Could you check a few things on this model? Use its own coordinates, in mm. Face numbers are marked on the shaded views. A direction names the side the tool comes from. Round coordinates to 2 decimals unless told otherwise and drop trailing zeros. Loops run counter-clockwise (first coordinate to the right, second up) from the corner with the lowest first, then second, coordinate; pieces in that order, holes last. Notation, with made-up numbers: M 76,20 L 115,20 A20 cw 115,43 Z; hole C 30,-22.5 d2. An arc over 180 degrees is marked long. Return JSON: item names as keys, results as strings. Group by question number.
```python
from build123d import *

# Parameters (mm, degrees)
BOSS_EXTRUDE1_DEPTH     = 20
FILLET1_R               = 2
SHELL1_T                = -4
CUT_EXTRUDE1_DEPTH      = 43.708313008
CUT_EXTRUDE1_DEPTH_BACK = 43.708313008
SKETCH2_R               = 5


with BuildPart() as part:
    # Sketch1 → Boss-Extrude1 (new body)
    with BuildSketch(Plane.XY):
        with BuildLine():
            Line((-30, 20), (30, 20))
            ThreePointArc((30, 20), (31.414213562, 19.414213562), (32, 18))
            Line((32, 18), (32, -18))
            ThreePointArc((32, -18), (31.414213562, -19.414213562), (30, -20))
            Line((30, -20), (-30, -20))
            ThreePointArc((-30, -20), (-31.414213562, -19.414213562), (-32, -18))
            Line((-32, -18), (-32, 18))
            ThreePointArc((-32, 18), (-31.414213562, 19.414213562), (-30, 20))
        make_face()
    extrude(amount=BOSS_EXTRUDE1_DEPTH)

    # Fillet1
    fillet1_edges = [part.edges().sort_by_distance(p)[0] for p in [
        (0, -20, 0),
        (-31.414213562, -19.414213562, 0),
        (-32, 0, 0),
        (-31.414213562, 19.414213562, 0),
        (0, 20, 0),
        (31.414213562, 19.414213562, 0),
        (32, 0, 0),
        (31.414213562, -19.414213562, 0),
    ]]
    fillet(fillet1_edges, radius=FILLET1_R)

    # Shell1
    shell1_openings = [part.faces().sort_by_distance(p)[0] for p in [
        (0, 0, 20),
    ]]
    offset(amount=SHELL1_T, openings=shell1_openings, kind=Kind.INTERSECTION)

    # Sketch2 → Cut-Extrude1 (cut, two sides: drawn at the far end of the back side and taken through both)
    with BuildSketch(Plane(origin=(0, 0, 0), x_dir=(1, 0, 0), z_dir=(0, 1, 0)).offset(-CUT_EXTRUDE1_DEPTH_BACK)):
        with Locations((-16, -20)):
            Circle(SKETCH2_R)
        with Locations((16, -20)):
            Circle(SKETCH2_R)
    extrude(amount=CUT_EXTRUDE1_DEPTH + CUT_EXTRUDE1_DEPTH_BACK, mode=Mode.SUBTRACT)


solid = part.part
```
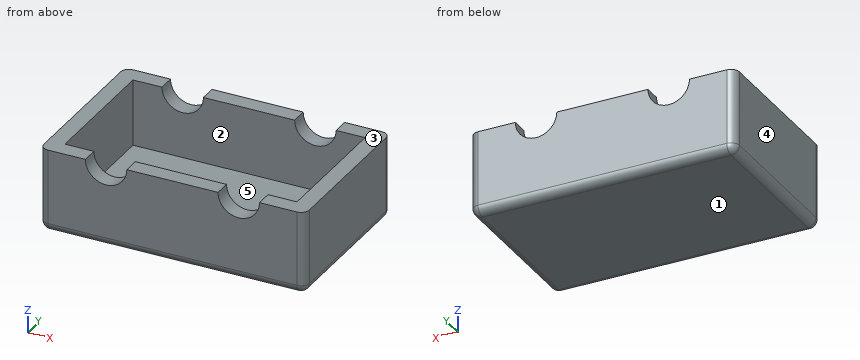
1. We'd pull the mould along X, two halves only. Please class the marked faces 3, 4 and 5: +X half, -X half, draft (parallel to the pull), parting line (faces both ways), or undercut.
2. I'm going to push a flat-ended pin straight in: pin 1 Ø9.5 at (x, y) = (-4, 1) entering from +Z. Where does the tip first touch, or does it pass through?
3. I need wall thicknesses on probe 1 along Y at (x, z) = (25, 14.25); probe 2 along X at (y, z) = (8, 7.25); probe 3 along X at (y, z) = (16.5, 17). Which ranges of each line are inside material? Lowest first, please.
4. On a 3-axis mill with a long thin cutter (end or side, diameter ignored), from which of +Z, -Z, +X, -X, +Y, -Y can I reach the whole of each face in a straight line? I mean the marked faces 1 and 2. Say none if no direction works.
5. If we section it at C-C, the plane x = 16: Please give me the cut outline in (y, z), then the cut area to 3 significant figures.
6. If we section it at A-A, the plane z = 10.5: Please give me the cut outline in (x, y).
7. If we section it at B-B, the plane y = 10.5: Please give me the cut outline in (x, z), then the cut area to 3 significant figures.
Geometry results:
{
 "1": {"face 3": "draft", "face 4": "-X half", "face 5": "undercut"},
 "2": {"pin 1": "z = 4"},
 "3": {"probe 1": "-20 to -16, 16 to 20", "probe 2": "-32 to -28, 28 to 32", "probe 3": "-32 to -20, -12 to 12, 20 to 32"},
 "4": {"face 1": "-Z, +X, -X, +Y, -Y", "face 2": "+Z"},
 "5": {"outline": "M -20,2 A2 ccw -18,0 L 18,0 A2 ccw 20,2 L 20,15 L 16,15 L 16,4 L -16,4 L -16,15 L -20,15 Z", "area": "246 mm^2"},
 "6": {"outline": "M -32,-18 A2 ccw -30,-20 L 30,-20 A2 ccw 32,-18 L 32,18 A2 ccw 30,20 L -30,20 A2 ccw -32,18 Z; hole M -28,-16 L 28,-16 L 28,16 L -28,16 Z"},
 "7": {"outline": "M -32,2 A2 ccw -30,0 L 30,0 A2 ccw 32,2 L 32,20 L 28,20 L 28,4 L -28,4 L -28,20 L -32,20 Z", "area": "382 mm^2"}
}
